```python
from build123d import *

# Parameters (mm, degrees)
SKETCH_1_W           = 45
SKETCH_1_H           = 15
EXTRUDE_1_DEPTH      = 2
SKETCH_2_W           = 3
SKETCH_2_H           = 3
EXTRUDE_2_DEPTH      = 1
EXTRUDE_3_DEPTH      = 2
EXTRUDE_3_DEPTH_BACK = 2
CUT_EXTRUDE_1_DEPTH  = 41.234344782
FILLET_1_R           = 0.2
FILLET_2_R           = 0.1


with BuildPart() as part:
    # 草图1 → 凸台-拉伸1 (new body)
    with BuildSketch(Plane.XY):
        Rectangle(SKETCH_1_W, SKETCH_1_H)
    extrude(amount=-EXTRUDE_1_DEPTH)

    # 草图2 → 凸台-拉伸2 (add)
    with BuildSketch(Plane.XY):
        with Locations((-15, 0)):
            Rectangle(SKETCH_2_W, SKETCH_2_H)
        with Locations((15, 0)):
            Rectangle(SKETCH_2_W, SKETCH_2_H)
    extrude(amount=EXTRUDE_2_DEPTH)

    # 草图3 → 凸台-拉伸3 (add, two sides: drawn at the far end of the back side and taken through both)
    with BuildSketch(Plane(origin=(0, 0, 0), x_dir=(1, 0, 0), z_dir=(0, 1, 0)).offset(-EXTRUDE_3_DEPTH_BACK)):
        with BuildLine():
            Line((-16.95, -2.5), (-13.05, -2.5))
            Line((-13.05, -2.5), (-13.05, -1.555590279))
            ThreePointArc((-13.05, -1.555590279), (-13.219957697, -1.088161527), (-13.5, -0.677124344))
            Line((-13.5, -0.677124344), (-16.5, -0.677124344))
            ThreePointArc((-16.5, -0.677124344), (-16.780042303, -1.088161527), (-16.95, -1.555590279))
            Line((-16.95, -1.555590279), (-16.95, -2.5))
        make_face()
        with BuildLine():
            Line((16.5, -0.677124344), (13.5, -0.677124344))
            ThreePointArc((13.5, -0.677124344), (13.219957697, -1.088161527), (13.05, -1.555590279))
            Line((13.05, -1.555590279), (13.05, -2.5))
            Line((13.05, -2.5), (16.95, -2.5))
            Line((16.95, -2.5), (16.95, -1.555590279))
            ThreePointArc((16.95, -1.555590279), (16.780042303, -1.088161527), (16.5, -0.677124344))
        make_face()
    extrude(amount=EXTRUDE_3_DEPTH + EXTRUDE_3_DEPTH_BACK)

    # 草图4 → 切除-拉伸1 (cut, through all)
    with BuildSketch(Plane.ZY.offset(16.95)):
        with BuildLine():
            Line((2.5, 1.95), (1.555590279, 1.95))
            ThreePointArc((1.555590279, 1.95), (1.088161527, 1.780042303), (0.677124344, 1.5))
            Line((0.677124344, 1.5), (0.677124344, 2))
            Line((0.677124344, 2), (2.5, 2))
            Line((2.5, 2), (2.5, 1.95))
        make_face()
        with BuildLine():
            Line((0.677124344, -2), (2.5, -2))
            Line((2.5, -2), (2.5, -1.95))
            Line((2.5, -1.95), (1.555590279, -1.95))
            ThreePointArc((1.555590279, -1.95), (1.088161527, -1.780042303), (0.677124344, -1.5))
            Line((0.677124344, -1.5), (0.677124344, -2))
        make_face()
    extrude(amount=-CUT_EXTRUDE_1_DEPTH, mode=Mode.SUBTRACT)

    # 圆角1
    fillet_1_edges = [part.edges().sort_by_distance(p)[0] for p in [
        (22.5, 0, -2),
        (0, 7.5, -2),
        (-22.5, 0, -2),
        (0, 7.5, 0),
        (22.5, 0, 0),
        (0, -7.5, 0),
        (-22.5, 0, 0),
        (0, -7.5, -2),
        (-22.5, 7.5, -1),
        (22.5, 7.5, -1),
        (22.5, -7.5, -1),
        (-22.5, -7.5, -1),
    ]]
    fillet(fillet_1_edges, radius=FILLET_1_R)

    # 圆角2
    fillet_2_edges = [part.edges().sort_by_distance(p)[0] for p in [
        (13.05, 0, 2.5),
        (16.95, 0, 2.5),
        (-16.95, 0, 2.5),
        (-13.05, 0, 2.5),
        (-15, -1.95, 2.5),
        (15, -1.95, 2.5),
        (-15, 1.95, 2.5),
        (15, 1.95, 2.5),
    ]]
    fillet(fillet_2_edges, radius=FILLET_2_R)


solid = part.part
```
The model under review builds one solid part; all positions refer to its coordinate system, in mm. A direction names the side the tool comes from. Round coordinates to 2 decimals unless told otherwise and drop trailing zeros. Loops run counter-clockwise (first coordinate to the right, second up) from the corner with the lowest first, then second, coordinate; pieces in that order, holes last. Notation, with made-up numbers: (-36, 26) -> (-21, 26) arc R29 ccw to (-21, 49) -> close; hole circle Ø6 at (16.5, 53). An arc over 180 degrees is marked (long way). Answer as a JSON object with one key per item and string values. Group by question number.
1) We need section B-B on x = -3.5. Write out the cut boundary in (y, z).
2) For faces 4 (the face through (14.97, 1.78, 1.09)), 5 (the face through (15, 1.95, 2)), 6 (the face through (14.97, -1.78, 1.09)), 7 (the face through (-16.777, -0.027, 1.082)), 8 (the face through (-13.22, -0.03, 1.09)), list the 3-axis set-ups (+Z, -Z, +X, -X, +Y, -Y) from which the entire face can be reached by the end or side of a thin tool; tool diameter is ignored.
3) For pin 1 Ø1.5 at (x, y) = (12.5, 3.5) entering from +Z; pin 2 Ø0.9 at (y, z) = (-0.5, 2) entering from -X; pin 3 Ø0.5 at (x, z) = (-15.5, 0) entering from -Y; pin 4 Ø0.7 at (x, z) = (14.5, 2) entering from -Y, all flat-tipped, find the tip position at first contact; note any pin that passes through.
4) We need section C-C on y = 2.5. Write out the cut boundary in (x, z), then the cut area to 3 significant figures.
5) We need section A-A on z = 2. Write out the cut boundary in (x, y), then the cut area to 3 significant figures.
6) For line 1 (X direction, y = 0.5, z = 0.45); line 2 (X direction, y = -1, z = 2.3); line 3 (Z direction, x = -3.5, y = 4.25), list the stretches that pass through material, from the lowest coordinate up. Write a range as [from, to].
7) Mouldability with a two-part tool opening along X and no side actions: class faces 1 (the face through (-15, 0, 2.5)), 2 (the face through (22.5, 0, -1)), 3 (the face through (13.223, -0.027, 1.082)) as released by +X, released by -X, zero draft, split by the parting line, or undercut.
Result set:
{
 "1": {"outline": "(-7.5, -1.8) arc R0.2 ccw to (-7.3, -2) -> (7.3, -2) arc R0.2 ccw to (7.5, -1.8) -> (7.5, -0.2) arc R0.2 ccw to (7.3, 0) -> (-7.3, 0) arc R0.2 ccw to (-7.5, -0.2) -> close"},
 "2": {"face 4": "+X, -X, +Y", "face 5": "+Z, +X, -X, +Y", "face 6": "+X, -X, -Y", "face 7": "-X, +Y, -Y", "face 8": "+Y, -Y"},
 "3": {"pin 1": "z = 0", "pin 2": "x = -16.95", "pin 3": "y = -7.5", "pin 4": "y = -1.95"},
 "4": {"outline": "(-22.5, -1.8) arc R0.2 ccw to (-22.3, -2) -> (22.3, -2) arc R0.2 ccw to (22.5, -1.8) -> (22.5, -0.2) arc R0.2 ccw to (22.3, 0) -> (-22.3, 0) arc R0.2 ccw to (-22.5, -0.2) -> close", "area": "90.0 mm²"},
 "5": {"outline": "(-16.95, -1.95) -> (-13.05, -1.95) -> (-13.05, 1.95) -> (-16.95, 1.95) -> close; (13.05, -1.95) -> (16.95, -1.95) -> (16.95, 1.95) -> (13.05, 1.95) -> close", "area": "30.4 mm²"},
 "6": {"line 1": "[-16.5, -13.5], [13.5, 16.5]", "line 2": "[-16.95, -13.05], [13.05, 16.95]", "line 3": "[-2, 0]"},
 "7": {"face 1": "zero draft", "face 2": "released by +X", "face 3": "undercut"}
}
